Work out the finished part from the listing and answer in its coordinate system (mm). A direction names the side the tool comes from. Give positions to 0.01 mm unless a question says otherwise; leave off trailing zeros. Loops run counter-clockwise (first coordinate to the right, second up) from the corner with the lowest first, then second, coordinate; pieces in that order, holes last.
```python
from build123d import *

# Parameters (mm, degrees)
SKETCH1_W           = 127
SKETCH1_H           = 107.95
BOSS_EXTRUDE1_DEPTH = 3.175
SKETCH2_W           = 3.302
SKETCH2_H           = 6.604
CUT_EXTRUDE1_DEPTH  = 84.400427157
SKETCH3_R           = 1.27
SKETCH3_W           = 3.377042817
SKETCH3_H           = 3.429
SKETCH3_W_2         = 3.429
SKETCH3_H_2         = 6.604
SKETCH3_W_3         = 5.08
SKETCH3_H_3         = 3.377042817
SKETCH3_W_4         = 10.414
CUT_EXTRUDE2_DEPTH  = 84.400427157
SKETCH4_W           = 25.4
SKETCH4_H           = 12.7
CUT_EXTRUDE3_DEPTH  = 84.400427157
SKETCH5_W           = 30.48
SKETCH5_H           = 17.475489296
CUT_EXTRUDE4_DEPTH  = 84.400427157
SKETCH6_W           = 30.48
SKETCH6_H           = 22.225
CUT_EXTRUDE5_DEPTH  = 84.400427157


with BuildPart() as part:
    # Sketch1 → Boss-Extrude1 (new body)
    with BuildSketch(Plane(origin=(0, 0, 0), x_dir=(1, 0, 0), z_dir=(0, 1, 0))):
        Rectangle(SKETCH1_W, SKETCH1_H)
    extrude(amount=BOSS_EXTRUDE1_DEPTH)

    # Sketch2 → Cut-Extrude1 (cut, through all)
    with BuildSketch(Plane.XZ):
        Polygon((-34.7345, 47.625), (-41.4655, 47.625), (-41.4655, 54.229), (-47.4345, 54.229), (-47.4345, 47.625), (-60.198, 47.625), (-63.5, 47.625), (-63.5, 54.229), (-63.5, 63.03162391), (63.5, 63.03162391), (63.5, 54.229), (63.5, 47.625), (60.198, 47.625), (47.4345, 47.625), (47.4345, 54.229), (41.4655, 54.229), (41.4655, 47.625), (34.7345, 47.625), (34.7345, 54.229), (28.7655, 54.229), (28.7655, 47.625), (22.0345, 47.625), (22.0345, 54.229), (16.0655, 54.229), (16.0655, 47.625), (9.3345, 47.625), (9.3345, 54.229), (3.3655, 54.229), (3.3655, 47.625), (-3.3655, 47.625), (-3.3655, 54.229), (-9.3345, 54.229), (-9.3345, 47.625), (-16.0655, 47.625), (-16.0655, 54.229), (-22.0345, 54.229), (-22.0345, 47.625), (-28.7655, 47.625), (-28.7655, 54.229), (-34.7345, 54.229), align=None)
        with Locations((61.849, 38.227)):
            Rectangle(SKETCH2_W, SKETCH2_H)
        with Locations((61.849, 25.527)):
            Rectangle(SKETCH2_W, SKETCH2_H)
        with Locations((61.849, 12.827)):
            Rectangle(SKETCH2_W, SKETCH2_H)
        with Locations((61.849, 0.127)):
            Rectangle(SKETCH2_W, SKETCH2_H)
        with Locations((61.849, -12.573)):
            Rectangle(SKETCH2_W, SKETCH2_H)
        with Locations((61.849, -25.273)):
            Rectangle(SKETCH2_W, SKETCH2_H)
        with Locations((61.849, -37.973)):
            Rectangle(SKETCH2_W, SKETCH2_H)
        with Locations((-61.849, -37.973)):
            Rectangle(SKETCH2_W, SKETCH2_H)
        with Locations((-61.849, -25.273)):
            Rectangle(SKETCH2_W, SKETCH2_H)
        with Locations((-61.849, -12.573)):
            Rectangle(SKETCH2_W, SKETCH2_H)
        with Locations((-61.849, 0.127)):
            Rectangle(SKETCH2_W, SKETCH2_H)
        with Locations((-61.849, 12.827)):
            Rectangle(SKETCH2_W, SKETCH2_H)
        with Locations((-61.849, 25.527)):
            Rectangle(SKETCH2_W, SKETCH2_H)
        with Locations((-61.849, 38.227)):
            Rectangle(SKETCH2_W, SKETCH2_H)
        with Locations((61.849, -50.673)):
            Rectangle(SKETCH2_W, SKETCH2_H)
        with Locations((-61.849, -50.673)):
            Rectangle(SKETCH2_W, SKETCH2_H)
    extrude(amount=-CUT_EXTRUDE1_DEPTH, mode=Mode.SUBTRACT)

    # Sketch3 → Cut-Extrude2 (cut, through all)
    with BuildSketch(Plane(origin=(0, 3.175, 0), x_dir=(1, 0, 0), z_dir=(0, 1, 0))):
        with Locations(Location((0, 3.175, 0), (0, 0, 270))):
            Circle(SKETCH3_R)
        with Locations((-36.538478592, -3.289010704)):
            Rectangle(SKETCH3_W, SKETCH3_H)
        with Locations((-36.5125, 10.998489296)):
            Rectangle(SKETCH3_W_2, SKETCH3_H_2)
        with Locations((-36.538478592, 3.060989296)):
            Rectangle(SKETCH3_W, SKETCH3_H)
        with Locations((-10.033, -9.639010705)):
            Rectangle(SKETCH3_W_3, SKETCH3_H_3)
        with Locations((-33.02, -9.639010705)):
            Rectangle(SKETCH3_W_4, SKETCH3_H_3)
        with Locations((-20.193, -9.639010705)):
            Rectangle(SKETCH3_W_3, SKETCH3_H_3)
        with Locations((0.127, -9.639010705)):
            Rectangle(SKETCH3_W_3, SKETCH3_H_3)
        with Locations((10.287, -9.639010705)):
            Rectangle(SKETCH3_W_3, SKETCH3_H_3)
        with Locations((20.447, -9.639010705)):
            Rectangle(SKETCH3_W_3, SKETCH3_H_3)
        with Locations((33.02, -9.639010705)):
            Rectangle(SKETCH3_W_4, SKETCH3_H_3)
        with Locations((36.538478592, -3.289010704)):
            Rectangle(SKETCH3_W, SKETCH3_H)
        with Locations((36.538478592, 3.060989296)):
            Rectangle(SKETCH3_W, SKETCH3_H)
        with Locations((36.5125, 10.998489296)):
            Rectangle(SKETCH3_W_2, SKETCH3_H_2)
    extrude(amount=-CUT_EXTRUDE2_DEPTH, mode=Mode.SUBTRACT)

    # Sketch4 → Cut-Extrude3 (cut, through all)
    with BuildSketch(Plane(origin=(0, 3.175, 0), x_dir=(1, 0, 0), z_dir=(0, 1, 0))):
        with Locations((0, 3.175)):
            Rectangle(SKETCH4_W, SKETCH4_H)
    extrude(amount=-CUT_EXTRUDE3_DEPTH, mode=Mode.SUBTRACT)

    # Sketch5 → Cut-Extrude4 (cut, through all)
    with BuildSketch(Plane(origin=(0, 3.175, 0), x_dir=(1, 0, 0), z_dir=(0, 1, 0))):
        with Locations((0.127, 0.787255352)):
            Rectangle(SKETCH5_W, SKETCH5_H)
    extrude(amount=-CUT_EXTRUDE4_DEPTH, mode=Mode.SUBTRACT)

    # Sketch6 → Cut-Extrude5 (cut, through all)
    with BuildSketch(Plane(origin=(0, 3.175, 0), x_dir=(1, 0, 0), z_dir=(0, 1, 0))):
        with Locations((0.127, 3.162010704)):
            Rectangle(SKETCH6_W, SKETCH6_H)
    extrude(amount=-CUT_EXTRUDE5_DEPTH, mode=Mode.SUBTRACT)


solid = part.part
```
Q1. Consider line 1 along X through (y, z) = (2.55, 3); line 2 along X through (y, z) = (0.4, -1); line 3 along Z through (x, y) = (-10, 0.55) (3 decimals). Determine where each line is inside the solid, lowest interval first.
Q2. Section A-A on x = -20.5 is taken. Give the vertices of the cut face in (y, z) (3 decimals), plus the area to 3 significant figures.
Q3. Determine the mould class of faces 6 (the face through (62, 2, 34.925)), 7 (the face through (60.198, 2, -25)), 8 (the face through (20, 2, 11.328)) for opening direction X: +X half, -X half, draft (parallel to the pull), parting line (faces both ways), or undercut.
Q4. Section B-B on z = 40 is taken. Give the vertices of the cut face in (x, y) (3 decimals).
Q5. Which of the six approach directions +Z, -Z, +X, -X, +Y, -Y give full straight-line access (tool end or side, diameter ignored) to faces 1 (the face through (-34.734, 2, 51)), 2 (the face through (-14, 2, 7.95)), 3 (the face through (-32, 2, 53.975)), 4 (the face through (60.198, 2, 0)), 5 (the face through (-62, 2, -28.575))?
Q6. Given pin 1 (1 mm diameter, centred on x = -62, y = 1, fed in from -Z); pin 2 (1 mm diameter, centred on y = 2, z = 50, fed in from +X); pin 3 (1.6 mm diameter, centred on x = 61.5, y = 1.5, fed in from +Z) (3 decimals), each flat-ended and moving along its own axis, determine where each tip first touches the part or whether it passes through.
Q7. Section C-C on y = 0.55 is taken. State how many separate pieces and enclosed holes the cut face has, plus the area to 3 significant figures.
Check result:
1. line 1: x = -60.2 to -38.23, -34.85 to -15.11, 15.37 to 34.85, 38.23 to 60.2
1. line 2: x = -60.2 to -15.11, 15.37 to 60.2
1. line 3: z = -53.975 to -14.275, 11.328 to 47.625
2. outline: (0, -53.975) - (3.175, -53.975) - (3.175, 7.95) - (0, 7.95) - close; (0, 11.328) - (3.175, 11.328) - (3.175, 53.975) - (0, 53.975) - close
2. area: 332 mm2
3. face 6: draft
3. face 7: +X half
3. face 8: undercut
4. outline: (-60.198, 0) - (60.198, 0) - (60.198, 3.175) - (-60.198, 3.175) - close
5. face 1: +Z, +Y, -Y
5. face 2: +Y, -Y
5. face 3: +Z, +X, -X, +Y, -Y
5. face 4: +X, +Y, -Y
5. face 5: -X, +Y, -Y
6. pin 1: stops at z = -47.37
6. pin 2: stops at x = 47.43
6. pin 3: stops at z = 47.625
7. separate pieces: 1
7. enclosed holes: 11
7. area: 11,900 mm2
